Source: CAD feature listing. Evaluate the final solid. Frame: model axes, mm. A direction names the side the tool comes from. Give positions to 0.01 mm unless a question says otherwise; leave off trailing zeros. Write each loop counter-clockwise with the first axis right and the second up, starting at its lowest first coordinate (ties: lowest second). Pieces come first, ordered by that corner, then holes. Notation, with made-up numbers: M -19,77.5 L 20,77.5 A20 ccw 20,94.5 Z; hole C 38,-8 d4. An arc over 180 degrees is marked long. Return JSON: item names as keys, results as strings.
```python
from build123d import *

# Parameters (mm, degrees)
PAD_DEPTH    = 16
SKETCH001_W  = 16
SKETCH001_H  = 300
PAD001_DEPTH = 16
SKETCH002_R  = 4
POCKET_DEPTH = 16.001


with BuildPart() as part:
    # Sketch → Pad (new body)
    with BuildSketch(Plane.YZ):
        Polygon((0, 0), (0, -100), (16, -100), (216, -100), (216, -84), (16, 300), (0, 300), align=None)
        Polygon((16, 265.363049), (197.959921, -84), (16, -84), align=None, mode=Mode.SUBTRACT)
    extrude(amount=PAD_DEPTH)

    # Sketch001 (on Face4 of Pad) → Pad001 (join)
    with BuildSketch(Plane(origin=(0, 0, 0), x_dir=(0, 1, 0), z_dir=(-1, 0, 0))):
        with Locations((8, -150)):
            Rectangle(SKETCH001_W, SKETCH001_H)
    extrude(amount=PAD001_DEPTH)

    # Sketch002 (on Face12 of Pad001) → Pocket (cut, through all)
    with BuildSketch(Plane.ZX.offset(16)):
        with Locations((50, -8)):
            Circle(SKETCH002_R)
        with Locations((160, -8)):
            Circle(SKETCH002_R)
    extrude(amount=-POCKET_DEPTH, mode=Mode.SUBTRACT)


solid = part.part
```
1) Draft query along Y for faces 5 (the face through (8, 216, -92)), 6 (the face through (-16, 8, 148)), 7 (the face through (0, 16, 111)), 8 (the face through (8, 108, -84)). Return one class per face: released by +Y, released by -Y, zero draft, split by the parting line, or undercut.
Numbers:
{"face 5": "released by +Y", "face 6": "zero draft", "face 7": "undercut", "face 8": "undercut"}
2) Cut plane C-C, the plane y = 64.5. Return the cut outline in (x, z).
Numbers:
{"outline": "M 0,-100 L 16,-100 L 16,-84 L 0,-84 Z; M 0,172.24 L 16,172.24 L 16,206.88 L 0,206.88 Z"}
3) Cut plane D-D, the plane z = 24.5. Return the cut outline in (x, y), then the cut area to 3 significant figures.
Numbers:
{"outline": "M -16,0 L 16,0 L 16,16 L -16,16 Z; M 0,141.45 L 16,141.45 L 16,159.49 L 0,159.49 Z", "area": "801 mm²"}
4) Line query: line 1 (X direction, y = 4.5, z = 50); line 2 (Y direction, x = -11, z = 12); line 3 (Z direction, x = 13, y = 182.5). Output: solid intervals per line, ascending. Write a range as [from, to].
Numbers:
{"line 1": "x = [-16, -12], [-4, 16]", "line 2": "y = [0, 16]", "line 3": "z = [-100, -84], [-54.32, -19.68]"}
5) Contact query for flat-ended pins moving along their axis: pin 1 Ø17.5 at (x, y) = (5, 71.5) entering from +Z; pin 2 Ø4 at (x, y) = (9.5, 86.5) entering from +Z; pin 3 Ø5 at (x, y) = (-10.5, 4.5) entering from -Z; pin 4 Ø8 at (x, z) = (-6, 223) entering from -Y. Output: stop coordinate, or through.
Numbers:
{"pin 1": "stops at z = 210.24", "pin 2": "stops at z = 168.48", "pin 3": "stops at z = 0", "pin 4": "stops at y = 0"}
6) Set-up query: faces 1 (the face through (7.888, 105.706, 93.127)), 2 (the face through (0, 139, 42)), 3 (the face through (7.89, 117.4, 105.31)), 4 (the face through (-8, 8, 0)). Return all of +Z, -Z, +X, -X, +Y, -Y with unobstructed straight access to the full face (end or side cutting, diameter ignored); none if empty.
Numbers:
{"face 1": "+X, -X", "face 2": "-Z, -X, +Y", "face 3": "+Z, +X, -X, +Y", "face 4": "-Z, -X, +Y, -Y"}
7) Cut plane A-A, the plane x = -8. Return the cut outline in (y, z).
Numbers:
{"outline": "M 0,0 L 16,0 L 16,46 L 0,46 Z; M 0,54 L 16,54 L 16,156 L 0,156 Z; M 0,164 L 16,164 L 16,300 L 0,300 Z"}
8) Cut plane B-B, the plane z = 160. Return the cut outline in (x, y), then the cut area to 3 significant figures.
Numbers:
{"outline": "M -16,0 L -12,0 L -12,16 L -16,16 Z; M -4,0 L 16,0 L 16,16 L -4,16 Z; M 0,70.88 L 16,70.88 L 16,88.92 L 0,88.92 Z", "area": "673 mm²"}
